The model under review builds one solid part; all positions refer to its coordinate system, in mm. Face numbers are marked on the shaded views. A direction names the side the tool comes from. Coordinates: 2 decimals unless noted, no trailing zeros. Loops run counter-clockwise (first coordinate to the right, second up) from the corner with the lowest first, then second, coordinate; pieces in that order, holes last. Notation, with made-up numbers: M 67,19.5 L 83,19.5 A25 ccw 83,42.5 Z; hole C 51.25,45 d4. An arc over 180 degrees is marked long. Use one line per item in the form item = value.
```python
from build123d import *

# Parameters (mm, degrees)
F2_R     = 5.715
F3_DEPTH = 13.463


with BuildPart() as f1:
    # F0 (on Front) → F1 (revolve)
    with BuildSketch(Plane.XZ):
        Polygon((0, 10.16), (0, 0), (13.462, 0), (13.462, 10.16), (10.668, 10.16), (10.668, 6.604), (3.81, 6.604), (3.81, 10.16), align=None)
    revolve(axis=Axis((6.731, 0, 0), (-1, 0, 0)))

    # F2 (on Right) → F3 (cut, through all)
    with BuildSketch(Plane.YZ):
        Circle(F2_R)
    extrude(amount=F3_DEPTH, mode=Mode.SUBTRACT)


solid = f1.part
```
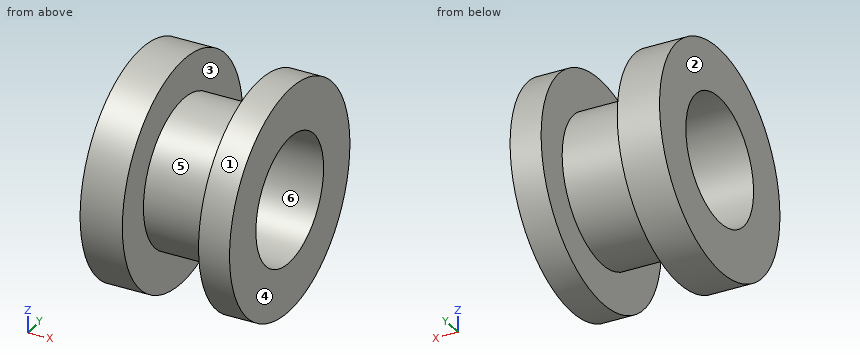
1. The part is to be moulded in two halves that separate along X. For the marked faces 1, 2, 3 and 4, say which applies: pulls with the +X half, pulls with the -X half, needs draft (parallel to the pull), parting line crosses it, or undercut.
Response values:
face_1 = needs draft
face_2 = pulls with the -X half
face_3 = undercut
face_4 = pulls with the +X half
2. Add section C-C (x = 5.75). State the section outline as (y, z) points (3 decimals), then the cut area to 3 significant figures.
Response values:
outline = C 0,0 d13.208; hole C 0,0 d11.43
area = 34.4 mm^2
3. Insertion check: P1, Ø3, axis at x = 6.5, y = 1.5, coming from the -Z side; P2, Ø4, axis at x = 5, z = -6, coming from the +Y side; P3, Ø3, axis at x = 4, y = -6.5, coming from the -Z side. Each pin has a flat end and moves straight along its axis. Give the tip position at first contact, or say it passes through.
Response values:
P1 = -6.6
P2 = 9.16
P3 = -8.84
4. Add section D-D (z = -8.25). State the section outline as (x, y) points, then the cut area to 3 significant figures.
Response values:
outline = M 0,-5.93 L 3.81,-5.93 L 3.81,5.93 L 0,5.93 Z; M 10.67,-5.93 L 13.46,-5.93 L 13.46,5.93 L 10.67,5.93 Z
area = 78.3 mm^2
5. Add section A-A (y = 0). State the section outline as (x, z) points (3 decimals).
Response values:
outline = M 0,-10.16 L 3.81,-10.16 L 3.81,-6.604 L 10.668,-6.604 L 10.668,-10.16 L 13.462,-10.16 L 13.462,-5.715 L 0,-5.715 Z; M 0,5.715 L 13.462,5.715 L 13.462,10.16 L 10.668,10.16 L 10.668,6.604 L 3.81,6.604 L 3.81,10.16 L 0,10.16 Z
6. Wall thickness on line 1 along X through (y, z) = (7.5, 5.5); line 2 along Y through (x, z) = (7, 0) (3 decimals); line 3 along Y through (x, z) = (3.5, 0) (3 decimals): over which ranges is each line inside the solid? List them lowest first. Write a range as from..to.
Response values:
line_1 = 0..3.81, 10.67..13.46
line_2 = -6.604..-5.715, 5.715..6.604
line_3 = -10.16..-5.715, 5.715..10.16
7. Machinability: for the marked faces 5 and 6, which of the approach directions +Z, -Z, +X, -X, +Y, -Y give a long, thin tool a straight path to every point of the face, cutting with its end or side? Answer none if there is none.
Response values:
face_5 = none
face_6 = +X, -X
